Read the model definition and answer for the solid it produces. Units are mm, in the model's axes. A direction names the side the tool comes from. Round coordinates to 2 decimals unless told otherwise and drop trailing zeros. Order: outer loops, then holes, each group sorted by start corner. A loop starts at its lowest first (then second) coordinate and runs counter-clockwise, first axis right, second up.
from build123d import *

# Parameters (mm, degrees)
BODY1_W                            = 5.9
BODY1_H                            = 4.5
EXTRUDE_1_DEPTH                    = 6
SKETCH_2_W                         = 4.7
SKETCH_2_H                         = 3.6
CUT_EXTRUDE_1_DEPTH                = 4.2
SKETCH_3_W                         = 5.9
SKETCH_3_H                         = 0.56
CUT_EXTRUDE_2_DEPTH                = 0.4
CHAMFER_1_SIZE                     = 0.35
CUT_EXTRUDE_3_REACH                = 11.543
SKETCH_4_W                         = 0.96
SKETCH_4_H                         = 1.98
SKETCH_5_W                         = 1.4
SKETCH_5_H                         = 0.2
CUT_EXTRUDE_4_DEPTH                = 10.54253635
SKETCH_7_W                         = 0.46
SKETCH_7_H                         = 1.77
CUT_EXTRUDE_5_DEPTH                = 0.1
CUT_EXTRUDE_6_REACH                = 11.543
SKETCH_8_W                         = 0.3
SKETCH_8_H                         = 4.2
CUT_EXTRUDE_7_REACH                = 11.543
SKETCH_15_W                        = 4.7
SKETCH_15_H                        = 1.95
CUT_EXTRUDE_9_DEPTH                = 0.65
CHAMFER_7_SIZE                     = 0.65
SKETCH_10_W                        = 0.5
SKETCH_10_H                        = 2.25
EXTRUDE_2_DEPTH                    = 0.3
CHAMFER_2_SIZE                     = 0.25
EXTRUDE_START                      = -4.9
SKETCH_12_W                        = 0.5
SKETCH_12_H                        = 0.5
EXTRUDE_4_DEPTH                    = 8.5
CHAMFER_3_SIZE                     = 0.1
CHAMFER_4_SIZE                     = 0.1
PATTERN_LINEAR_2_COUNT             = 2
PATTERN_LINEAR_2_PITCH             = 2
CHAMFER_3_OF_PATTERN_LINEAR_2_SIZE = 0.1
CHAMFER_4_OF_PATTERN_LINEAR_2_SIZE = 0.1
SKETCH_16_R                        = 0.05
CUT_EXTRUDE_10_DEPTH               = 3.4


with BuildPart() as part:
    # Body1 → Бобышка-Вытянуть1 (new body)
    with BuildSketch(Plane(origin=(0, 0, 0), x_dir=(1, 0, 0), z_dir=(0, 1, 0))):
        with Locations((2.95, -2.25)):
            Rectangle(BODY1_W, BODY1_H)
    extrude(amount=EXTRUDE_1_DEPTH)

    # Эскиз2 → Вырез-Вытянуть1 (cut)
    with BuildSketch(Plane(origin=(0, 6, 0), x_dir=(1, 0, 0), z_dir=(0, 1, 0))):
        with Locations((2.95, -2.25)):
            Rectangle(SKETCH_2_W, SKETCH_2_H)
    extrude(amount=-CUT_EXTRUDE_1_DEPTH, mode=Mode.SUBTRACT)

    # Эскиз3 → Вырез-Вытянуть2 (cut)
    with BuildSketch(Plane.XY.offset(4.5)):
        with Locations((2.95, 1.1)):
            Rectangle(SKETCH_3_W, SKETCH_3_H)
    extrude(amount=-CUT_EXTRUDE_2_DEPTH, mode=Mode.SUBTRACT)

    # Фаска1
    chamfer_1_edges = [part.edges().sort_by_distance(p)[0] for p in [
        (2.95, 6, 4.05),
        (5.3, 6, 2.25),
        (2.95, 6, 0.45),
        (0.6, 6, 2.25),
    ]]
    chamfer(chamfer_1_edges, length=CHAMFER_1_SIZE)

    # Эскиз4 → Вырез-Вытянуть3 (cut, up to next)
    with BuildSketch(Plane.XY.offset(4.5), mode=Mode.PRIVATE) as cut_extrude_3_sk1:
        with Locations((1.25, 3.24)):
            Rectangle(SKETCH_4_W, SKETCH_4_H)
    cut_extrude_3_tool1 = extrude(cut_extrude_3_sk1.sketch, amount=-CUT_EXTRUDE_3_REACH, mode=Mode.PRIVATE) & part.part
    # Эскиз4 → Вырез-Вытянуть3 (cut, up to next)
    with BuildSketch(Plane.XY.offset(4.5), mode=Mode.PRIVATE) as cut_extrude_3_sk2:
        with Locations((4.65, 3.24)):
            Rectangle(SKETCH_4_W, SKETCH_4_H)
    cut_extrude_3_tool2 = extrude(cut_extrude_3_sk2.sketch, amount=-CUT_EXTRUDE_3_REACH, mode=Mode.PRIVATE) & part.part
    add(cut_extrude_3_tool1.solids().sort_by_distance((1.25, 3.24, 4.5))[0], mode=Mode.SUBTRACT)
    add(cut_extrude_3_tool2.solids().sort_by_distance((4.65, 3.24, 4.5))[0], mode=Mode.SUBTRACT)

    # Эскиз5 → Вырез-Вытянуть4 (cut, through all)
    with BuildSketch(Plane.XY.offset(4.5)):
        with Locations((1.95, 0.1)):
            Rectangle(SKETCH_5_W, SKETCH_5_H)
    cut_extrude_4 = extrude(amount=-CUT_EXTRUDE_4_DEPTH, mode=Mode.SUBTRACT)

    # Эскиз7 → Вырез-Вытянуть5 (cut)
    with BuildSketch(Plane.XY.offset(4.5)):
        with Locations((4.4, 5.115)):
            Rectangle(SKETCH_7_W, SKETCH_7_H)
    extrude(amount=-CUT_EXTRUDE_5_DEPTH, mode=Mode.SUBTRACT)

    # Эскиз8 → Вырез-Вытянуть6 (cut, up to next)
    with BuildSketch(Plane.XY.offset(4.5), mode=Mode.PRIVATE) as cut_extrude_6_sk1:
        with Locations((2.95, 3.9)):
            Rectangle(SKETCH_8_W, SKETCH_8_H)
    cut_extrude_6_tool1 = extrude(cut_extrude_6_sk1.sketch, amount=-CUT_EXTRUDE_6_REACH, mode=Mode.PRIVATE) & part.part
    add(cut_extrude_6_tool1.solids().sort_by_distance((2.95, 3.9, 4.5))[0], mode=Mode.SUBTRACT)

    # Эскиз9 → Вырез-Вытянуть7 (cut, up to next)
    with BuildSketch(Plane.ZY, mode=Mode.PRIVATE) as cut_extrude_7_sk1:
        with BuildLine():
            Line((2.12, 6), (3.12, 6))
            Line((3.12, 6), (3.12, 4.5))
            ThreePointArc((3.12, 4.5), (2.62, 4), (2.12, 4.5))
            Line((2.12, 4.5), (2.12, 6))
        make_face()
    cut_extrude_7_tool1 = extrude(cut_extrude_7_sk1.sketch, amount=-CUT_EXTRUDE_7_REACH, mode=Mode.PRIVATE) & part.part
    cut_extrude_7 = cut_extrude_7_tool1.solids().sort_by_distance((0, 5.05036, 2.62))[0]
    add(cut_extrude_7, mode=Mode.SUBTRACT)

    # Зеркальное отражение1: Вырез-Вытянуть7 across plane
    add(cut_extrude_7.mirror(Plane(origin=(2.95, 0, 0), x_dir=(0, 0, 1), z_dir=(1, 0, 0))), mode=Mode.SUBTRACT)

    # Эскиз15 → Вырез-Вытянуть9 (cut)
    with BuildSketch(Plane(origin=(0, 1.8, 0), x_dir=(1, 0, 0), z_dir=(0, 1, 0))):
        with Locations((2.95, -1.425)):
            Rectangle(SKETCH_15_W, SKETCH_15_H)
    extrude(amount=-CUT_EXTRUDE_9_DEPTH, mode=Mode.SUBTRACT)

    # Фаска7
    chamfer_7_edges = [part.edges().sort_by_distance(p)[0] for p in [
        (2.95, 1.15, 2.4),
    ]]
    chamfer(chamfer_7_edges, length=CHAMFER_7_SIZE - 0.0001)  # a hair under: the kernel refuses the full size

    # Эскиз10 → Бобышка-Вытянуть2 (add)
    with BuildSketch(Plane.XY.offset(0.45)):
        with Locations((2.95, 2.275)):
            Rectangle(SKETCH_10_W, SKETCH_10_H)
    extrude(amount=EXTRUDE_2_DEPTH)

    # Фаска2
    chamfer_2_edges = [part.edges().sort_by_distance(p)[0] for p in [
        (2.95, 3.4, 0.75),
    ]]
    chamfer(chamfer_2_edges, length=CHAMFER_2_SIZE)

    # Эскиз12 → Бобышка-Вытянуть4 (add)
    with BuildSketch(Plane.XZ.offset(-0.2).offset(EXTRUDE_START)):
        with Locations((1.95, 2.8)):
            Rectangle(SKETCH_12_W, SKETCH_12_H)
    extrude_4 = extrude(amount=EXTRUDE_4_DEPTH)

    # Фаска3
    chamfer_3_edges = [part.edges().sort_by_distance(p)[0] for p in [
        (1.7, -3.4, 2.8),
        (1.95, -3.4, 2.55),
        (2.2, -3.4, 2.8),
        (1.95, -3.4, 3.05),
    ]]
    chamfer(chamfer_3_edges, length=CHAMFER_3_SIZE)

    # Фаска4
    chamfer_4_edges = [part.edges().sort_by_distance(p)[0] for p in [
        (1.7, 5.1, 2.8),
        (1.95, 5.1, 2.55),
        (2.2, 5.1, 2.8),
        (1.95, 5.1, 3.05),
    ]]
    chamfer(chamfer_4_edges, length=CHAMFER_4_SIZE)

    # Линейный массив2: Вырез-Вытянуть4, Бобышка-Вытянуть4 ×2
    with Locations(*[(i * PATTERN_LINEAR_2_PITCH, 0, 0) for i in range(1, PATTERN_LINEAR_2_COUNT)]):
        add(cut_extrude_4, mode=Mode.SUBTRACT)
        add(extrude_4)

    # Фаска3 of Линейный массив2
    chamfer_3_of_pattern_linear_2_edges = [part.edges().sort_by_distance(p)[0] for p in [
        (3.7, -3.4, 2.8),
        (3.95, -3.4, 2.55),
        (4.2, -3.4, 2.8),
        (3.95, -3.4, 3.05),
    ]]
    chamfer(chamfer_3_of_pattern_linear_2_edges, length=CHAMFER_3_OF_PATTERN_LINEAR_2_SIZE)

    # Фаска4 of Линейный массив2
    chamfer_4_of_pattern_linear_2_edges = [part.edges().sort_by_distance(p)[0] for p in [
        (3.7, 5.1, 2.8),
        (3.95, 5.1, 2.55),
        (4.2, 5.1, 2.8),
        (3.95, 5.1, 3.05),
    ]]
    chamfer(chamfer_4_of_pattern_linear_2_edges, length=CHAMFER_4_OF_PATTERN_LINEAR_2_SIZE)

    # Эскиз16 → Вырез-Вытянуть10 (cut)
    with BuildSketch(Plane.XZ):
        with Locations((1.95, 2.8)):
            Circle(SKETCH_16_R)
    extrude(amount=CUT_EXTRUDE_10_DEPTH, mode=Mode.SUBTRACT)


solid = part.part
Q1. For a pull along Z with two mould halves and no side action, classify faces 3 (the face through (3, 1.8, 3)), 4 (the face through (3, 3, 0)), 5 (the face through (4, 4, 4.05)), 6 (the face through (1, 0, 2)) as released by +Z, released by -Z, zero draft, split by the parting line, or undercut.
Outcome:
face 3: undercut
face 4: released by -Z
face 5: undercut
face 6: zero draft
Q2. For faces 1 (the face through (3, 4, 0.45)), 2 (the face through (5.9, 3, 2)), determine the directions among +Z, -Z, +X, -X, +Y, -Y from which every point of the face is accessible in a straight line to the end or side of a thin tool.
Outcome:
face 1: +Y
face 2: +Z, -Z, +X, +Y, -Y
Q3. A cutting plane is placed at B-B, the plane z = 1.2. Give the vertices of the cut face in (x, y), plus the area to 3 significant figures.
Outcome:
outline: (0, 0) - (1.25, 0) - (1.25, 0.2) - (2.65, 0.2) - (2.65, 0) - (3.25, 0) - (3.25, 0.2) - (4.65, 0.2) - (4.65, 0) - (5.9, 0) - (5.9, 6) - (5.65, 6) - (5.3, 5.65) - (5.3, 1.15) - (0.6, 1.15) - (0.6, 5.65) - (0.25, 6) - (0, 6) - close
area: 11.9 mm2
Q4. Straight lines are drawn through the part: probe 1 along X at (y, z) = (3.25, 4.25); probe 2 along X at (y, z) = (2.5, 2.6); probe 3 along X at (y, z) = (1.5, 1.4). For each, find the intervals that lie inside material, in ascending order.
Outcome:
probe 1: x = 0 to 0.77, 1.73 to 2.8, 3.1 to 4.17, 5.13 to 5.9
probe 2: x = 0 to 0.6, 1.7 to 2.2, 3.7 to 4.2, 5.3 to 5.9
probe 3: x = 0 to 0.6, 5.3 to 5.9
Q5. Flat-ended cylindrical pins translate along their axes: pin 1 (1.8 mm diameter, centred on x = 4.5, y = 3, fed in from -Z); pin 2 (0.6 mm diameter, centred on y = -2, z = 3, fed in from -X); pin 3 (0.5 mm diameter, centred on x = 5, z = 4, fed in from +Y). Find the tip coordinate at first contact, or state that the pin passes through.
Outcome:
pin 1: stops at z = 0
pin 2: stops at x = 1.7
pin 3: stops at y = 5.85
